Part print with two shaded views. Sizes in mm from the minimum x, y, z corner. A direction names the side the tool comes from. Coordinates: 2 decimals unless noted, no trailing zeros. Order: outer loops, then holes, each group sorted by start corner. A loop starts at its lowest first (then second) coordinate and runs counter-clockwise, first axis right, second up. Notation, with made-up numbers: (31, 30) - (84, 30) arc R6 ccw to (84, 35) - close; hole circle Ø10 at (62, 83.25). An arc over 180 degrees is marked (long way). One line per item, written item: value.
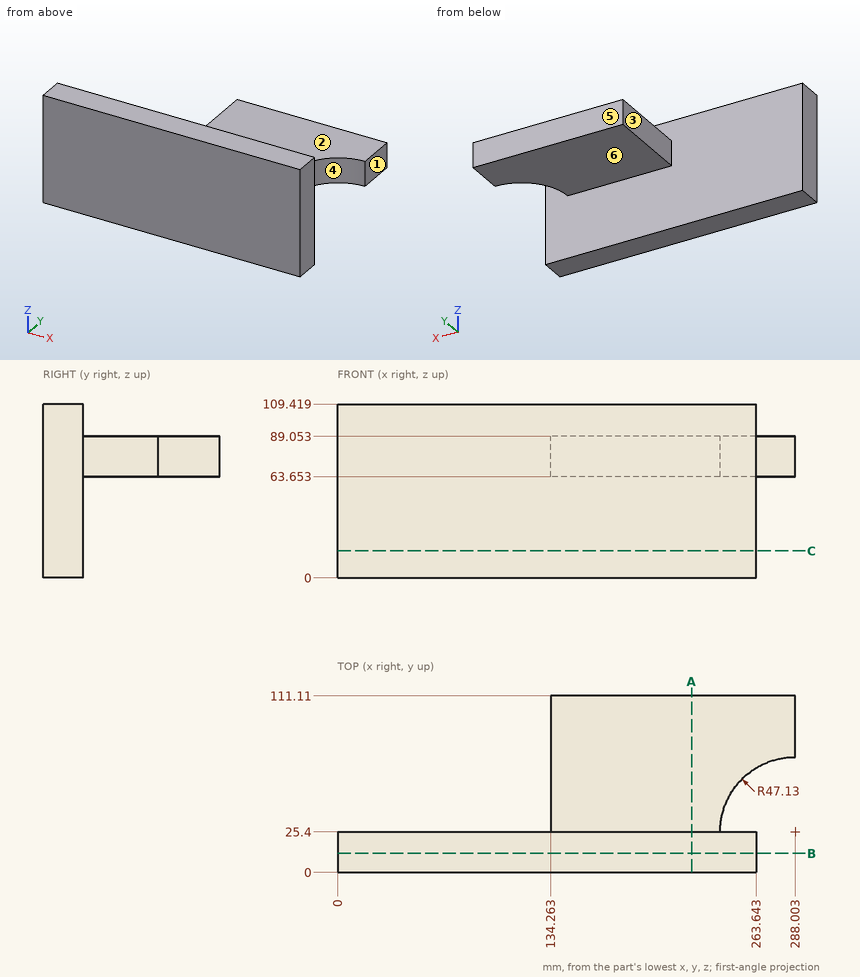
1. Band-saw the part on C-C, the plane z = 17. Give the cut face in (x, y), and give its area (3 significant figures).
Values found:
outline: (0, 0) - (263.64, 0) - (263.64, 25.4) - (0, 25.4) - close
area: 6,700 mm2
2. Band-saw the part on A-A, the plane x = 223. Give the cut face in (y, z).
Values found:
outline: (0, 0) - (25.4, 0) - (25.4, 63.65) - (111.11, 63.65) - (111.11, 89.05) - (25.4, 89.05) - (25.4, 109.42) - (0, 109.42) - close
3. Flat gauge pins, fed straight in: P1, Ø20.5, axis at y = 71.5, z = 80, coming from the -X side; P2, Ø2, axis at x = 95, z = 27.5, coming from the +Y side; P3, Ø7.5, axis at y = 18.5, z = 69.5, coming from the +X side. Where does each tip first touch, or does it go through?
Values found:
P1: stops at x = 134.26
P2: stops at y = 25.4
P3: stops at x = 263.64
4. Two-plate mould, pull along Y, no slides. Class the marked faces 4, 5 and 6: pulls with the +Y half, pulls with the -Y half, needs draft (parallel to the pull), parting line crosses it, or undercut.
Values found:
face 4: undercut
face 5: pulls with the +Y half
face 6: needs draft
5. Band-saw the part on B-B, the plane y = 12. Give the cut face in (x, z).
Values found:
outline: (0, 0) - (263.64, 0) - (263.64, 109.42) - (0, 109.42) - close
6. 3-axis set-ups, long thin cutter, end or side, ignore diameter. For the marked faces 1, 2 and 3: which of +Z, -Z, +X, -X, +Y, -Y reach the whole face in a straight line?
Values found:
face 1: +Z, -Z, +X, +Y, -Y
face 2: +Z, +X, -X, +Y
face 3: +Z, -Z, -X, +Y
7. Probe line 1 along X through (y, z) = (17, 70); line 2 along Y through (x, z) = (199.5, 51); line 3 along Z through (x, y) = (146.5, 50.5). List the from-to ranges inside material, lowest first.
Values found:
line 1: x = 0 to 263.64
line 2: y = 0 to 25.4
line 3: z = 63.65 to 89.05
